from build123d import *

# Parameters (mm, degrees)
BOSS_EXTRUDE1_DEPTH = 5.715
BOSS_EXTRUDE2_DEPTH = 29.21
SKETCH3_W           = 66.200858932
SKETCH3_H           = 4.6355
CUT_EXTRUDE1_DEPTH  = 31.75
SKETCH4_R           = 4.445
BOSS_EXTRUDE3_DEPTH = 14.605
SKETCH5_R           = 1.27
CUT_EXTRUDE2_DEPTH  = 7.62


with BuildPart() as part:
    # Sketch1 → Boss-Extrude1 (new body)
    with BuildSketch(Plane.XY):
        Polygon((41.275, 44.914422768), (36.195, 57.15), (-36.195, 57.15), (-41.275, 44.914422768), (-41.275, -44.914422768), (-36.195, -57.15), (36.195, -57.15), (41.275, -44.914422768), align=None)
    extrude(amount=BOSS_EXTRUDE1_DEPTH)

    # Sketch2 → Boss-Extrude2 (add)
    with BuildSketch(Plane.XY.offset(5.715)):
        Polygon((-41.275, 44.914422768), (-41.275, -44.914422768), (-36.195, -57.15), (36.195, -57.15), (41.275, -44.914422768), (41.275, 44.914422768), (36.195, 57.15), (-36.195, 57.15), align=None)
        Polygon((-33.100429466, 52.5145), (-36.6395, 43.99037188), (-36.6395, -43.99037188), (-33.100429466, -52.5145), (33.100429466, -52.5145), (36.6395, -43.99037188), (36.6395, 43.99037188), (33.100429466, 52.5145), align=None, mode=Mode.SUBTRACT)
    extrude(amount=BOSS_EXTRUDE2_DEPTH)

    # Sketch3 → Cut-Extrude1 (cut)
    with BuildSketch(Plane.XY.offset(34.925)):
        with Locations((0, 54.83225)):
            Rectangle(SKETCH3_W, SKETCH3_H)
    cut_extrude1 = extrude(amount=-CUT_EXTRUDE1_DEPTH, mode=Mode.SUBTRACT)

    # Mirror1: Cut-Extrude1 across plane
    add(cut_extrude1.mirror(Plane.ZX), mode=Mode.SUBTRACT)

    # Sketch4 → Boss-Extrude3 (add)
    with BuildSketch(Plane.XY.offset(5.715)):
        with Locations((22.225, -31.75)):
            Circle(SKETCH4_R)
        with Locations((-22.225, -31.75)):
            Circle(SKETCH4_R)
        with Locations((22.225, 31.75)):
            Circle(SKETCH4_R)
        with Locations((-22.225, 31.75)):
            Circle(SKETCH4_R)
    extrude(amount=BOSS_EXTRUDE3_DEPTH)

    # Sketch5 → Cut-Extrude2 (cut)
    with BuildSketch(Plane.XY.offset(20.32)):
        with Locations((-22.225, 31.75)):
            Circle(SKETCH5_R)
        with Locations((22.225, 31.75)):
            Circle(SKETCH5_R)
        with Locations((22.225, -31.75)):
            Circle(SKETCH5_R)
        with Locations((-22.225, -31.75)):
            Circle(SKETCH5_R)
    extrude(amount=-CUT_EXTRUDE2_DEPTH, mode=Mode.SUBTRACT)


solid = part.part
The model under review builds one solid part; all positions refer to its coordinate system, in mm. A direction names the side the tool comes from. Give positions to 0.01 mm unless a question says otherwise; leave off trailing zeros. Loops run counter-clockwise (first coordinate to the right, second up) from the corner with the lowest first, then second, coordinate; pieces in that order, holes last. Notation, with made-up numbers: (-7, 10.5) -> (23, 10.5) arc R33 cw to (23, 38.5) -> close; hole circle Ø5 at (15, -3). An arc over 180 degrees is marked (long way). Answer as a JSON object with one key per item and string values. Group by question number.
Q1. Take a section at B-B (y = -31.75). Write out the cut boundary in (x, z) (1 decimal).
Q2. Tool access review of faces 4 (the flat face through (21, 31, 20.32)), 5 (the flat face through (34.845, -48.312, 20.116)), 6 (the flat face through (0, -55, 3.175)), 7 (the flat face through (0, 57.15, 3)): name each direction out of +Z, -Z, +X, -X, +Y, -Y from which nothing blocks a thin tool from reaching the whole face with its end or side.
Q3. Take a section at D-D (y = -48). Write out the cut boundary in (x, z) (3 decimals).
Q4. Insertion check: pin 1 (2.5 mm diameter, centred on x = 24.5, y = -32, fed in from +Z); pin 2 (0.8 mm diameter, centred on x = 22, y = -31.5, fed in from +Z); pin 3 (2.5 mm diameter, centred on x = 13, y = -56, fed in from +Z) (3 decimals). Each pin has a flat end and moves straight along its axis. Give the tip position at first contact, or say it passes through.
Q5. Draft analysis for pull direction X (two halves, no side actions). For faces 1 (the flat face through (-38.7, 51.12, 17.22)), 2 (the flat face through (-1, 1, 0)), 3 (the flat face through (0, -52.514, 4)), state which applies: pulls with the +X half, pulls with the -X half, needs draft (parallel to the pull), parting line crosses it, or undercut.
Q6. Wall thickness on line 1 along X through (y, z) = (-18.5, 17) (1 decimal); line 2 along Z through (x, y) = (24.5, -25.5) (3 decimals); line 3 along X through (y, z) = (-31, 18) (1 decimal): over which ranges is each line inside the solid? List them lowest first.
Q7. Take a section at A-A (z = 8.5). State how many separate pieces and enclosed holes the cut face has, plus the area to 3 significant figures.
Answer below:
{
 "1": {"outline": "(-41.3, 0) -> (41.3, 0) -> (41.3, 34.9) -> (36.6, 34.9) -> (36.6, 5.7) -> (26.7, 5.7) -> (26.7, 20.3) -> (23.5, 20.3) -> (23.5, 12.7) -> (21, 12.7) -> (21, 20.3) -> (17.8, 20.3) -> (17.8, 5.7) -> (-17.8, 5.7) -> (-17.8, 20.3) -> (-21, 20.3) -> (-21, 12.7) -> (-23.5, 12.7) -> (-23.5, 20.3) -> (-26.7, 20.3) -> (-26.7, 5.7) -> (-36.6, 5.7) -> (-36.6, 34.9) -> (-41.3, 34.9) -> close"},
 "2": {"face 4": "+Z, +Y, -Y", "face 5": "+Z", "face 6": "+Z, -Y", "face 7": "+Z, -Z, +X, -X, +Y"},
 "3": {"outline": "(-39.994, 0) -> (39.994, 0) -> (39.994, 34.925) -> (34.975, 34.925) -> (34.975, 5.715) -> (-34.975, 5.715) -> (-34.975, 34.925) -> (-39.994, 34.925) -> close"},
 "4": {"pin 1": "stops at z = 20.32", "pin 2": "stops at z = 12.7", "pin 3": "stops at z = 3.175"},
 "5": {"face 1": "pulls with the -X half", "face 2": "needs draft", "face 3": "undercut"},
 "6": {"line 1": "x = -41.3 to -36.6, 36.6 to 41.3", "line 2": "z = 0 to 5.715", "line 3": "x = -41.3 to -36.6, -26.6 to -23.2, -21.2 to -17.8, 17.8 to 21.2, 23.2 to 26.6, 36.6 to 41.3"},
 "7": {"separate pieces": "6", "enclosed holes": "0", "area": "1,310 mm2"}
}
